from build123d import *

# Parameters (mm, degrees)
F0_W     = 127
F0_H     = 60
F1_DEPTH = 3
F3_DEPTH = 3
F5_DEPTH = 3


with BuildPart() as f1:
    # F0 (on Front) → F1 (new body)
    with BuildSketch(Plane.XZ):
        Rectangle(F0_W, F0_H)
    extrude(amount=F1_DEPTH)

    # F2 (on face) → F3 (join, through all)
    with BuildSketch(Plane.XZ.offset(3)):
        Polygon((-3, 30), (0, 30), (3, 30), (3, 33), (0, 33), (-3, 33), align=None)
        Polygon((9, 30), (12, 30), (15, 30), (15, 33), (12, 33), (9, 33), align=None)
        Polygon((21, 30), (24, 30), (27, 30), (27, 33), (24, 33), (21, 33), align=None)
        Polygon((33, 30), (36, 30), (39, 30), (39, 33), (36, 33), (33, 33), align=None)
        Polygon((45, 30), (48, 30), (51, 30), (51, 33), (48, 33), (45, 33), align=None)
        Polygon((57, 30), (60, 30), (63, 30), (63, 33), (60, 33), (57, 33), align=None)
        Polygon((-36, 30), (-33, 30), (-33, 33), (-36, 33), (-39, 33), (-39, 30), align=None)
        Polygon((-63, 30), (-60, 30), (-57, 30), (-57, 33), (-60, 33), (-63, 33), align=None)
        Polygon((-45, 30), (-45, 33), (-48, 33), (-51, 33), (-51, 30), (-48, 30), align=None)
        Polygon((-27, 30), (-24, 30), (-21, 30), (-21, 33), (-24, 33), (-27, 33), align=None)
        Polygon((-15, 30), (-12, 30), (-9, 30), (-9, 33), (-12, 33), (-15, 33), align=None)
        Polygon((-9, -33), (-9, -30), (-12, -30), (-15, -30), (-15, -33), (-12, -33), align=None)
        Polygon((36, -30), (33, -30), (33, -33), (36, -33), (39, -33), (39, -30), align=None)
        Polygon((63, -30), (60, -30), (57, -30), (57, -33), (60, -33), (63, -33), align=None)
        Polygon((45, -30), (45, -33), (48, -33), (51, -33), (51, -30), (48, -30), align=None)
        Polygon((-36, -30), (-39, -30), (-39, -33), (-36, -33), (-33, -33), (-33, -30), align=None)
        Polygon((-57, -30), (-60, -30), (-63, -30), (-63, -33), (-60, -33), (-57, -33), align=None)
        Polygon((-51, -30), (-51, -33), (-48, -33), (-45, -33), (-45, -30), (-48, -30), align=None)
        Polygon((27, -30), (24, -30), (21, -30), (21, -33), (24, -33), (27, -33), align=None)
        Polygon((15, -30), (12, -30), (9, -30), (9, -33), (12, -33), (15, -33), align=None)
        Polygon((3, -30), (0, -30), (-3, -30), (-3, -33), (0, -33), (3, -33), align=None)
        Polygon((-27, -30), (-27, -33), (-24, -33), (-21, -33), (-21, -30), (-24, -30), align=None)
    extrude(amount=-F3_DEPTH)

    # F4 (on face) → F5 (join, through all)
    with BuildSketch(Plane.XZ.offset(3)):
        Polygon((-63.5, -3), (-63.5, 0), (-63.5, 3), (-66.5, 3), (-66.5, 0), (-66.5, -3), align=None)
        Polygon((-63.5, 9), (-63.5, 12), (-63.5, 15), (-66.5, 15), (-66.5, 12), (-66.5, 9), align=None)
        Polygon((-63.5, 21), (-63.5, 24), (-63.5, 27), (-66.5, 27), (-66.5, 24), (-66.5, 21), align=None)
        Polygon((-63.5, -24), (-63.5, -21), (-66.5, -21), (-66.5, -24), (-66.5, -27), (-63.5, -27), align=None)
        Polygon((-63.5, -15), (-63.5, -12), (-63.5, -9), (-66.5, -9), (-66.5, -12), (-66.5, -15), align=None)
        Polygon((66.5, 24), (66.5, 27), (63.5, 27), (63.5, 24), (63.5, 21), (66.5, 21), align=None)
        Polygon((63.5, -9), (63.5, -12), (63.5, -15), (66.5, -15), (66.5, -12), (66.5, -9), align=None)
        Polygon((63.5, -24), (63.5, -27), (66.5, -27), (66.5, -24), (66.5, -21), (63.5, -21), align=None)
        Polygon((66.5, 12), (66.5, 15), (63.5, 15), (63.5, 12), (63.5, 9), (66.5, 9), align=None)
        Polygon((63.5, 0), (63.5, -3), (66.5, -3), (66.5, 0), (66.5, 3), (63.5, 3), align=None)
    extrude(amount=-F5_DEPTH)


solid = f1.part
Geometry check sheet. Reference: the model listing, model coordinates, mm. A direction names the side the tool comes from. Round coordinates to 2 decimals unless told otherwise and drop trailing zeros. Write each loop counter-clockwise with the first axis right and the second up, starting at its lowest first coordinate (ties: lowest second). Pieces come first, ordered by that corner, then holes. Notation, with made-up numbers: (10.25, -0.75) - (69.25, -0.75) arc R9 cw to (69.25, 8.25) - close; hole circle Ø5 at (38.25, 44). An arc over 180 degrees is marked (long way). One line per item, written item: value.
1. Set-up check for faces 4 (the face through (27, -2, 31)), 5 (the face through (-65, -2, 27)), 6 (the face through (-65, -2, 3)): record each of +Z, -Z, +X, -X, +Y, -Y from which the full face is reachable in a straight line by a thin tool's end or side.
The answers:
face 4: +Z, +Y, -Y
face 5: +Z, -X, +Y, -Y
face 6: -X, +Y, -Y
2. Mould release check, pull along X, two halves, no side actions. Record for faces 1 (the face through (-21, -2, -32)), 2 (the face through (24, -2, -33)), 3 (the face through (63.5, -1, 28)): released by +X, released by -X, zero draft, split by the parting line, or undercut.
The answers:
face 1: undercut
face 2: zero draft
face 3: released by +X
3. Depth check by flat-ended pin: pin 1 Ø1.5 at (x, y) = (55, -1.5) entering from -Z; pin 2 Ø0.9 at (y, z) = (-1, -32) entering from +X; pin 3 Ø1.5 at (y, z) = (-1, 32) entering from -X. Enter the tip coordinate at first touch or a pass-through.
The answers:
pin 1: stops at z = -30
pin 2: stops at x = 63
pin 3: stops at x = -63
4. Cross-section at A-A on z = -7. Record the boundary of the cut face in (x, y).
The answers:
outline: (-63.5, -3) - (63.5, -3) - (63.5, 0) - (-63.5, 0) - close
5. Scan lines: L1, parallel to X at y = -1.7, z = 5.5; L2, parallel to Z at x = 5.5, y = -2.45. Record each from-to range of solid material in increasing order.
The answers:
L1: x = -63.5 to 63.5
L2: z = -30 to 30
6. Cross-section at B-B on x = -30.5. Record the boundary of the cut face in (y, z).
The answers:
outline: (-3, -30) - (0, -30) - (0, 30) - (-3, 30) - close
